Design review of the part built by this model. Coordinates are the model's own, in mm. A direction names the side the tool comes from. Coordinates: 2 decimals unless noted, no trailing zeros. Write each loop counter-clockwise with the first axis right and the second up, starting at its lowest first coordinate (ties: lowest second). Pieces come first, ordered by that corner, then holes. Notation, with made-up numbers: M 15.5,55 L 46.5,55 A31 cw 46.5,84 Z; hole C 56.5,-16.5 d4. An arc over 180 degrees is marked long. Return JSON: item names as keys, results as strings. Group by question number.
```python
from build123d import *

# Parameters (mm, degrees)
SKETCH_R            = 1.1
SKETCH_R_2          = 1.5
PAD_DEPTH           = 3
BOX_W               = 3
BOX_H               = 3
BOX_DEPTH           = 5
BOX_PLACEMENT_ANGLE = 27


with BuildPart() as body:
    # Sketch → Pad (new body)
    with BuildSketch(Plane.XY):
        Polygon((-5.660254, -27.124356), (3, -32.124356), (20, -2.679492), (20, 22.320508), (10, 22.320508), (10, 0), align=None)
        with Locations((15, 17.320508)):
            Circle(SKETCH_R, mode=Mode.SUBTRACT)
        with Locations((1.169873, -25.294229)):
            Circle(SKETCH_R, mode=Mode.SUBTRACT)
        with Locations((14.687408, -1.255987)):
            Circle(SKETCH_R_2, mode=Mode.SUBTRACT)
    extrude(amount=PAD_DEPTH)


with BuildPart() as fusion:
    # Box → Box (new body)
    with BuildSketch(Plane.XY):
        with Locations((1.5, 1.5)):
            Rectangle(BOX_W, BOX_H)
    extrude(amount=BOX_DEPTH)


with BuildPart() as fusion_1:
    # Box placement: moved
    add(fusion.part.moved(Location((1, -11, 0))).rotate(Axis((1, -11, 0), (0, 0, -1)), BOX_PLACEMENT_ANGLE))

    # Fusion: union Body
    add(body.part)


solid = fusion_1.part
```
Item 1: The part is to be moulded in two halves that separate along Y. For faces 5 (the flat face through (15, 22.321, 1)), 6 (the flat face through (10, -5, 3)), 7 (the flat face through (11.38, -17.61, 1.48)), 8 (the cylindrical face through (1.027, -24.204, 1.479)), say which applies: pulls with the +Y half, pulls with the -Y half, needs draft (parallel to the pull), parting line crosses it, or undercut.
Item 2: For pin 1 (3.5 mm diameter, centred on x = 15, y = 17.32, fed in from +Z); pin 2 (1 mm diameter, centred on y = -14.5, z = 1, fed in from +X); pin 3 (3 mm diameter, centred on y = -12.5, z = 2, fed in from +X), all flat-tipped, find the tip position at first contact; note any pin that passes through.
Item 3: Add section A-A (x = 15). Write out the cut boundary in (y, z), plus the area to 3 significant figures.
Item 4: Add section D-D (y = 14). Write out the cut boundary in (x, z), plus the area to 3 significant figures.
Item 5: Machinability: for faces 1 (the flat face through (4.344, -11.044, 3.986)), 2 (the flat face through (10, 11, 1)), 3 (the flat face through (-1.246, -19.478, 1.479)), 4 (the flat face through (3, -10, 5)), which of the approach directions +Z, -Z, +X, -X, +Y, -Y give a long, thin tool a straight path to every point of the face, cutting with its end or side? Answer none if there is none.
Item 6: Add section B-B (z = 1). Write out the cut boundary in (x, y), plus the area to 3 significant figures.
Item 7: Add section C-C (z = 3.6). Write out the cut boundary in (x, y) (3 decimals), plus the area to 3 significant figures.
Item 8: For line 1 (Y direction, x = 15, z = 0.85); line 2 (Z direction, x = 14.5, y = 9); line 3 (X direction, y = 5.5, z = 2.05), list the stretches that pass through material, from the lowest coordinate up.
Geometry check:
{
 "1": {"face 5": "pulls with the +Y half", "face 6": "needs draft", "face 7": "pulls with the -Y half", "face 8": "undercut"},
 "2": {"pin 1": "z = 3", "pin 2": "x = 13.46", "pin 3": "x = 15.2"},
 "3": {"outline": "M -11.34,0 L -2.72,0 L -2.72,3 L -11.34,3 Z; M 0.21,0 L 16.22,0 L 16.22,3 L 0.21,3 Z; M 18.42,0 L 22.32,0 L 22.32,3 L 18.42,3 Z", "area": "85.6 mm^2"},
 "4": {"outline": "M 10,0 L 20,0 L 20,3 L 10,3 Z", "area": "30.0 mm^2"},
 "5": {"face 1": "+Z, +X, -Y", "face 2": "+Z, -Z, -X, +Y", "face 3": "+Z, -Z, -X", "face 4": "+Z, +X, -X, +Y, -Y"},
 "6": {"outline": "M -5.66,-27.12 L 3,-32.12 L 20,-2.68 L 20,22.32 L 10,22.32 L 10,0 L 4.55,-9.44 L 2.36,-8.33 L 1,-11 L 3.05,-12.04 Z; hole C 1.17,-25.29 d2.2; hole C 14.69,-1.26 d3; hole C 15,17.32 d2.2", "area": "556 mm^2"},
 "7": {"outline": "M 1,-11 L 3.673,-12.362 L 5.035,-9.689 L 2.362,-8.327 Z", "area": "9.00 mm^2"},
 "8": {"line 1": "-11.34 to -2.72, 0.21 to 16.22, 18.42 to 22.32", "line 2": "0 to 3", "line 3": "10 to 20"}
}
